Here's how the part is built. I have some questions about the finished solid (model axes, mm). Face numbers are marked on the shaded views. A direction names the side the tool comes from. Coordinates: 2 decimals unless noted, no trailing zeros. Loops run counter-clockwise (first coordinate to the right, second up) from the corner with the lowest first, then second, coordinate; pieces in that order, holes last. Notation, with made-up numbers: (-13.5, -20) -> (31.5, -20) arc R9 ccw to (31.5, -9) -> close; hole circle Ø4 at (58.5, 11). An arc over 180 degrees is marked (long way). Answer as a JSON object with one key per item and string values. Group by question number.
Q1. I want a section at D-D on x = -7. Write out the boundary of the cut face in (y, z), then the cut area to 3 significant figures.
Q2. I'm going to push flat-ended pins straight in: pin 1 (1 mm diameter, centred on x = 16.06, y = 9.12, fed in from +Z); pin 2 (1.5 mm diameter, centred on y = -2.88, z = 2.5, fed in from -X); pin 3 (6 mm diameter, centred on x = -9.44, y = 8.12, fed in from -Z); pin 4 (3 mm diameter, centred on y = 9.62, z = 2.5, fed in from +X). Where does each tip first touch, or does it pass through?
Q3. I need wall thicknesses on line 1 (X direction, y = 4.25, z = 3.5); line 2 (Y direction, x = 4, z = 0.5); line 3 (X direction, y = 3.5, z = 0.3). Which ranges of each line are inside material? Lowest first, please.
Q4. I want a section at B-B on z = 0.45. Write out the boundary of the cut face in (x, y).
Q5. I want a section at C-C on y = 0.5. Write out the boundary of the cut face in (x, z), then the cut area to 3 significant figures.
Q6. On a 3-axis mill with a long thin cutter (end or side, diameter ignored), from which of +Z, -Z, +X, -X, +Y, -Y can I reach the whole of each face in a straight line? I mean the marked faces 4, 5, 6 and 7. Say none if no direction works.
Q7. Thinking about a two-plate mould opening in Y: for the marked faces 1, 2 and 3, which applies, released by +Y, released by -Y, zero draft, split by the parting line, or undercut?
Q8. I want a section at A-A on x = 7. Write out the boundary of the cut face in (y, z), then the cut area to 3 significant figures.
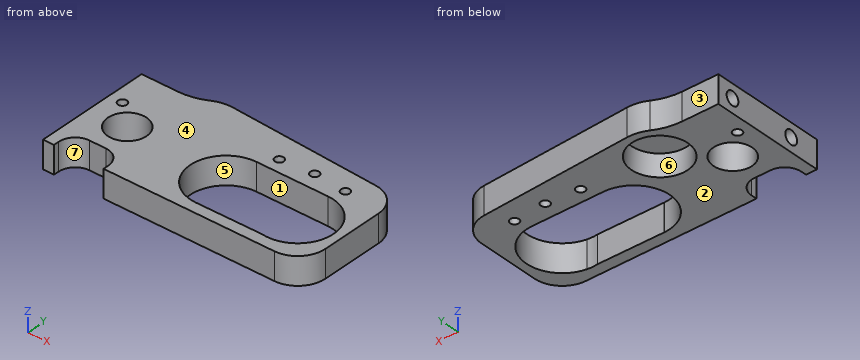
```python
from build123d import *

# Parameters (mm, degrees)
SKETCH1_R           = 0.8
SKETCH1_R_2         = 3.5
SKETCH1_R_3         = 5.1
BOSS_EXTRUDE1_DEPTH = 5
SKETCH2_R           = 1.25
CUT_EXTRUDE1_DEPTH  = 5
BOSS_EXTRUDE2_START = -1
SKETCH21_R          = 5.1
BOSS_EXTRUDE2_DEPTH = 1
SKETCH22_W          = 9
SKETCH22_H          = 4
CUT_EXTRUDE2_DEPTH  = 10
FILLET1_R           = 3


with BuildPart() as part:
    # Sketch1 → Boss-Extrude1 (new body)
    with BuildSketch(Plane(origin=(0, 0, 0), x_dir=(0, 1, 0), z_dir=(0, 0, 1))):
        with BuildLine():
            ThreePointArc((7.923715338, -23.061842121), (11.348253353, -21.704991773), (12.914157128, -18.370857874))
            Line((12.914157128, -18.370857874), (14.611258571, 9.036437401))
            ThreePointArc((14.611258571, 9.036437401), (14.470096631, 10.842810788), (13.835805455, 12.540039768))
            ThreePointArc((13.835805455, 12.540039768), (12.931450551, 14.850335933), (12.623684243, 17.312165753))
            Line((12.623684243, 17.312165753), (12.623684243, 23.938157879))
            Line((12.623684243, 23.938157879), (-8.376315757, 23.938157879))
            Line((-8.376315757, 23.938157879), (-8.376315757, -18.061842121))
            ThreePointArc((-8.376315757, -18.061842121), (-6.911849663, -21.597376027), (-3.376315757, -23.061842121))
            Line((-3.376315757, -23.061842121), (7.923715338, -23.061842121))
        make_face()
        with BuildLine():
            Line((-6.37591859, -2.133696229), (-6.376315757, -2.061842121))
            ThreePointArc((-6.376315757, -2.061842121), (0.123684243, 4.438157879), (6.623684243, -2.061842121))
            Line((6.623684243, -2.061842121), (6.623684243, -15.061842121))
            ThreePointArc((6.623684243, -15.061842121), (0.625179068, -21.542467318), (-6.298932046, -16.061842121))
            ThreePointArc((-6.298932046, -16.061842121), (-6.376216465, -15.097769724), (-6.309594086, -14.132901895))
            Line((-6.309594086, -14.132901895), (-6.37591859, -2.133696229))
        make_face(mode=Mode.SUBTRACT)
        with Locations(Location((9.123684243, -16.061842121, 0), (0, 0, 270))):
            Circle(SKETCH1_R, mode=Mode.SUBTRACT)
        with Locations(Location((9.623684243, -10.061842121, 0), (0, 0, 270))):
            Circle(SKETCH1_R, mode=Mode.SUBTRACT)
        with Locations(Location((9.123684243, -4.061842121, 0), (0, 0, 270))):
            Circle(SKETCH1_R, mode=Mode.SUBTRACT)
        with Locations(Location((1.537022692, 17.094912388, 0), (0, 0, 270))):
            Circle(SKETCH1_R_2, mode=Mode.SUBTRACT)
        with Locations(Location((8.123684243, 9.438157879, 0), (0, 0, 270))):
            Circle(SKETCH1_R_3, mode=Mode.SUBTRACT)
        with Locations(Location((5.623684243, 21.438157879, 0), (0, 0, 270))):
            Circle(SKETCH1_R, mode=Mode.SUBTRACT)
    extrude(amount=BOSS_EXTRUDE1_DEPTH)

    # Sketch2 → Cut-Extrude1 (cut)
    with BuildSketch(Plane(origin=(-23.938157879, 0, 0), x_dir=(0, -1, 0), z_dir=(-1, 0, 0))):
        with Locations(Location((-9.623684243, 2.5, 0), (0, 0, 90))):
            Circle(SKETCH2_R)
        with Locations(Location((2.876315757, 2.5, 0), (0, 0, 90))):
            Circle(SKETCH2_R)
    extrude(amount=-CUT_EXTRUDE1_DEPTH, mode=Mode.SUBTRACT)

    # Sketch21 → Boss-Extrude2 (add)
    with BuildSketch(Plane.XY.offset(5).offset(BOSS_EXTRUDE2_START)):
        with Locations((-9.438157879, 8.123684243)):
            Circle(SKETCH21_R)
    extrude(amount=BOSS_EXTRUDE2_DEPTH)

    # Sketch22 → Cut-Extrude2 (cut)
    with BuildSketch(Plane(origin=(0, 0, 0), x_dir=(1, 0, 0), z_dir=(0, 0, -1))):
        with Locations((-17.438157879, 6.376315757)):
            Rectangle(SKETCH22_W, SKETCH22_H)
    extrude(amount=-CUT_EXTRUDE2_DEPTH, mode=Mode.SUBTRACT)

    # Fillet1
    fillet1_edges = [part.edges().sort_by_distance(p)[0] for p in [
        (-12.938157879, -4.376315757, 2.5),
        (-21.938157879, -4.376315757, 2.5),
    ]]
    fillet(fillet1_edges, radius=FILLET1_R)


solid = part.part
```
Result set:
{
 "1": {"outline": "(-8.38, 0) -> (3.64, 0) -> (3.64, 4) -> (12.6, 4) -> (12.6, 0) -> (14.49, 0) -> (14.49, 5) -> (-8.38, 5) -> close", "area": "78.5 mm²"},
 "2": {"pin 1": "passes through", "pin 2": "stops at x = -18.94", "pin 3": "stops at z = 4", "pin 4": "stops at x = 23.06"},
 "3": {"line 1": "x = -23.94 to -19.31, -14.88 to -12.76, -6.12 to -2.96, 20.08 to 23.06", "line 2": "y = -8.38 to -6.37, 6.62 to 8.33, 9.92 to 13.8", "line 3": "x = -23.94 to -19.99, -14.2 to -11.59, -7.29 to -3.49, 20.62 to 23.06"},
 "4": {"outline": "(-23.94, -8.38) -> (-21.94, -8.38) -> (-21.94, -7.38) arc R3 cw to (-18.94, -4.38) -> (-15.94, -4.38) arc R3 cw to (-12.94, -7.38) -> (-12.94, -8.38) -> (18.06, -8.38) arc R5 ccw to (23.06, -3.38) -> (23.06, 7.92) arc R5 ccw to (18.37, 12.91) -> (-9.04, 14.61) arc R6.5 ccw to (-12.54, 13.84) arc R10 cw to (-17.31, 12.62) -> (-23.94, 12.62) -> close; hole circle Ø1.6 at (-21.44, 5.62); hole circle Ø7 at (-17.09, 1.54); hole circle Ø10.2 at (-9.44, 8.12); hole (2.06, -6.38) -> (14.13, -6.31) arc R6.5 ccw (long way) to (15.06, 6.62) -> (2.06, 6.62) arc R6.5 ccw to start; hole circle Ø1.6 at (4.06, 9.12); hole circle Ø1.6 at (10.06, 9.62); hole circle Ø1.6 at (16.06, 9.12)"},
 "5": {"outline": "(-23.94, 0) -> (-20.44, 0) -> (-20.44, 5) -> (-23.94, 5) -> close; (-13.75, 0) -> (-4.43, 0) -> (-4.43, 5) -> (-13.75, 5) -> close; (21.55, 0) -> (23.06, 0) -> (23.06, 5) -> (21.55, 5) -> close", "area": "71.7 mm²"},
 "6": {"face 4": "+Z, +X, -X, +Y, -Y", "face 5": "+Z, -Z", "face 6": "-Z", "face 7": "+Z, -Z, -Y"},
 "7": {"face 1": "undercut", "face 2": "zero draft", "face 3": "released by +Y"},
 "8": {"outline": "(-8.38, 0) -> (-6.35, 0) -> (-6.35, 5) -> (-8.38, 5) -> close; (6.62, 0) -> (13.62, 0) -> (13.62, 5) -> (6.62, 5) -> close", "area": "45.1 mm²"}
}
